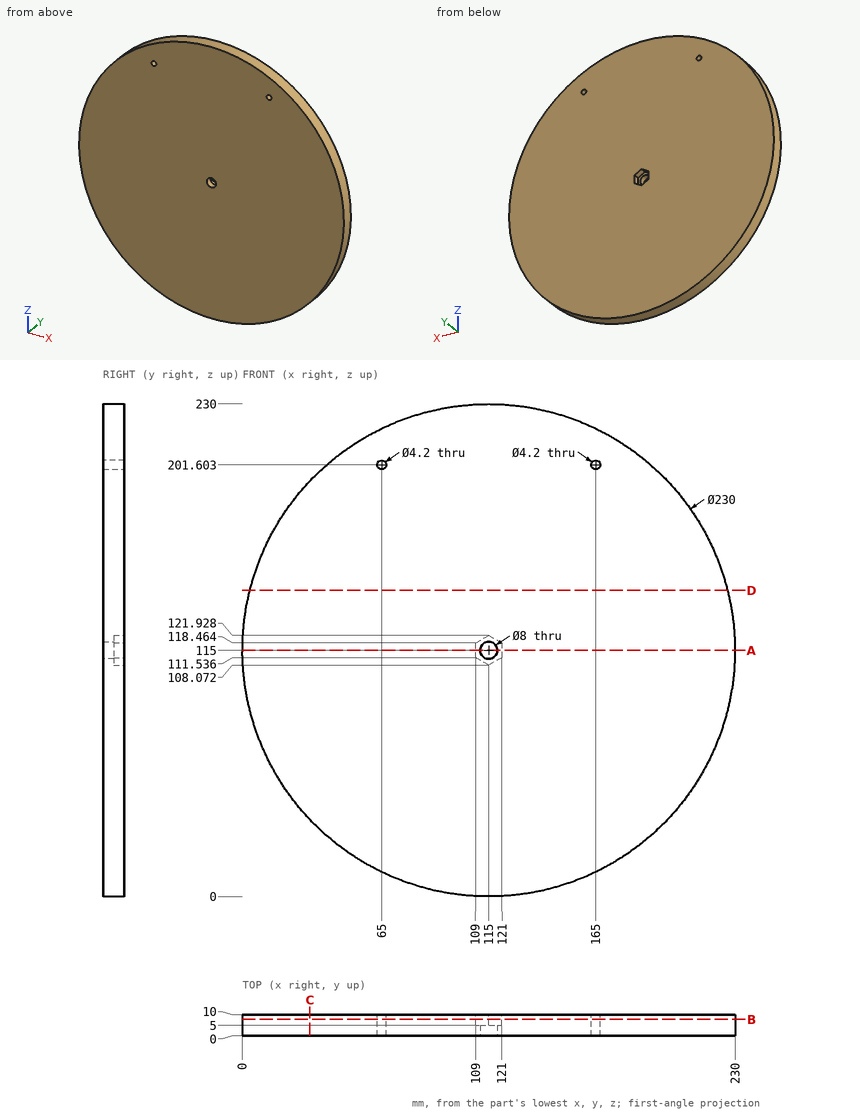
Verification items for this drawing (mm, ordinates from the low corner). Coordinates: 2 decimals unless noted, no trailing zeros. Order: outer loops, then holes, each group sorted by start corner. A loop starts at its lowest first (then second) coordinate and runs counter-clockwise, first axis right, second up.
Q1. Sectioned sample at B-B on y = 7.75. Record the cut outline in (x, z) (1 decimal).
Reply:
outline: circle Ø230 at (115, 115); hole circle Ø4.2 at (65, 201.6); hole (109, 111.5) - (115, 108.1) - (121, 111.5) - (121, 118.5) - (115, 121.9) - (109, 118.5) - close; hole circle Ø4.2 at (165, 201.6)
Q2. Sectioned sample at C-C on x = 31.5. Record the cut outline in (y, z) (1 decimal).
Reply:
outline: (0, 35.9) - (10, 35.9) - (10, 194.1) - (0, 194.1) - close
Q3. Sectioned sample at D-D on z = 143. Record the cut outline in (x, y).
Reply:
outline: (3.46, 0) - (226.54, 0) - (226.54, 10) - (3.46, 10) - close
Q4. Thickness scan on probe 1 along Z at (x, y) = (112.5, 4) (1 decimal); probe 2 along Z at (x, y) = (165, 5.75); probe 3 along X at (y, z) = (4.5, 79.5). Record the ranges inside material, lowest first.
Reply:
probe 1: z = 0 to 111.9, 118.1 to 230
probe 2: z = 11.44 to 199.5, 203.7 to 218.56
probe 3: x = 5.62 to 224.38
Q5. Sectioned sample at A-A on z = 115. Record the cut outline in (x, y), and give its area (3 significant figures).
Reply:
outline: (0, 0) - (111, 0) - (111, 5) - (109, 5) - (109, 10) - (0, 10) - close; (119, 0) - (230, 0) - (230, 10) - (121, 10) - (121, 5) - (119, 5) - close
area: 2,200 mm2
Q6. Depth check by flat-ended pin: pin 1 Ø1 at (y, z) = (6, 25.5) entering from +X; pin 2 Ø5 at (x, y) = (57.5, 3.5) entering from +Z (1 decimal); pin 3 Ø5 at (x, y) = (92.5, 8.5) entering from +Z. Enter the tip coordinate at first touch or a pass-through.
Reply:
pin 1: stops at x = 187.83
pin 2: stops at z = 216
pin 3: stops at z = 228.25
